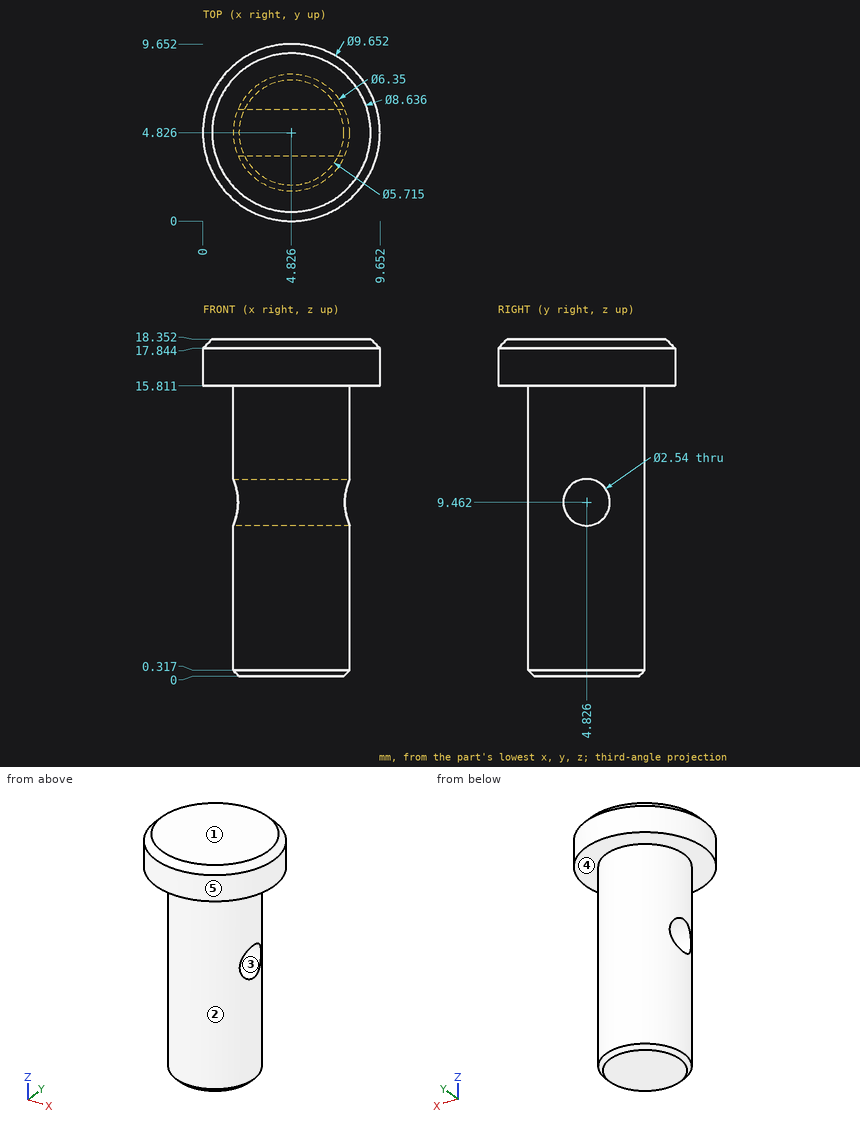
Input: dimensioned drawing with shaded views. Units: mm. Origin: part minimum x, y, z. A direction names the side the tool comes from. Coordinates: 2 decimals unless noted, no trailing zeros. One line per item, written item: value.
(1) Pin query (flat end, axial travel): pin 1 (3.5 mm diameter, centred on y = 4.83, z = 9.46, fed in from +X); pin 2 (2 mm diameter, centred on x = 8, y = 8, fed in from +Z); pin 3 (3 mm diameter, centred on y = 2, z = 11.5, fed in from -X); pin 4 (4 mm diameter, centred on x = 1.5, z = 2.5, fed in from -Y). Return the tip coordinate at first contact, or that it passes through.
Filled in:
pin 1: x = 8
pin 2: z = 18.35
pin 3: x = 1.94
pin 4: y = 1.94
(2) Reachability of the marked faces 1 and 2 from +Z, -Z, +X, -X, +Y, -Y: full face, straight path, thin tool, end or side. Return the list, or none.
Filled in:
face 1: +Z, +X, -X, +Y, -Y
face 2: -Z
(3) Pull-direction query (Y, two-part tool) for the marked faces 3, 4 and 5; classes: +Y half, -Y half, draft (parallel to the pull), parting line (faces both ways), or undercut.
Filled in:
face 3: undercut
face 4: draft
face 5: parting line
(4) Line query: line 1 along Z through (x, y) = (3, 8.5); line 2 along Z through (x, y) = (5.5, 4.75); line 3 along X through (y, z) = (5, 3) (1 decimal). Output: solid intervals per line, ascending. Write a range as from..to.
Filled in:
line 1: 15.81..18.35
line 2: 0..8.19, 10.73..18.35
line 3: 1.7..8
